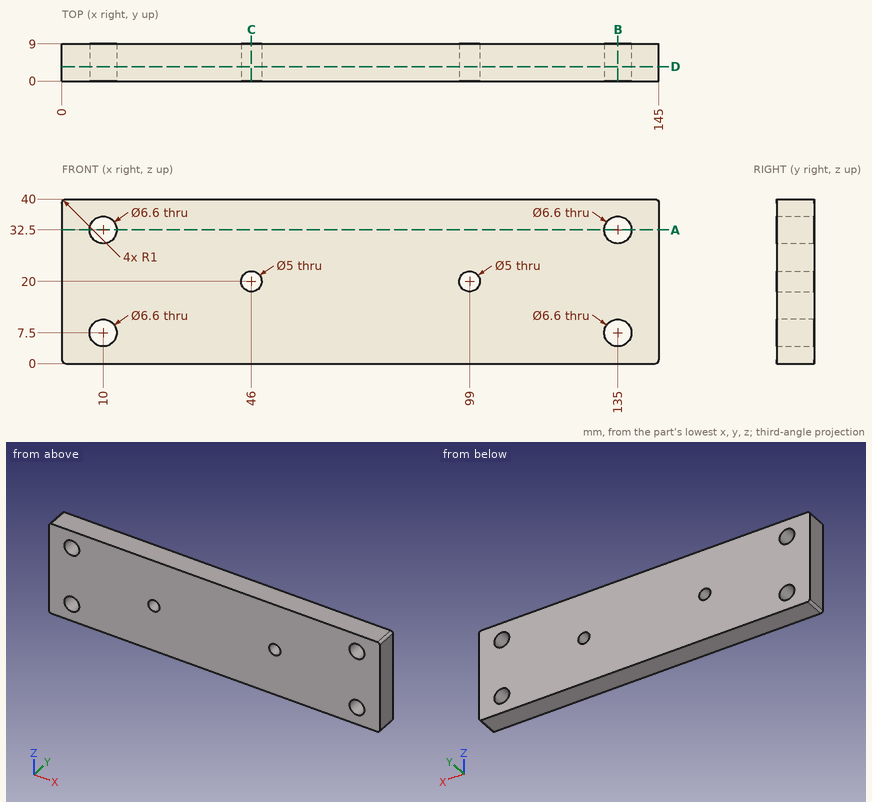
Source: three-view drawing plus pictorial views. Frame: mm from the lowest corner of the part. Give positions to 0.01 mm unless a question says otherwise; leave off trailing zeros. Order: outer loops, then holes, each group sorted by start corner. A loop starts at its lowest first (then second) coordinate and runs counter-clockwise, first axis right, second up. Notation, with made-up numbers: M 75.5,55 L 133.5,55 A23 cw 133.5,92 Z; hole C 4.5,72 d10. An arc over 180 degrees is marked long. One line per question, with ' | ' between items. Start each with the question number.
1. Section query B-B (x = 135). Return the cut outline in (y, z).
2. Section query C-C (x = 46). Return the cut outline in (y, z).
3. Material intervals for probe 1 along X at (y, z) = (3, 7.5); probe 2 along Z at (x, y) = (135, 3.5); probe 3 along X at (y, z) = (4.25, 20), sorted ascending. Write a range as [from, to].
4. Section query A-A (z = 32.5). Return the cut outline in (x, y), and give its area (3 significant figures).
5. Section query D-D (y = 3.5). Return the cut outline in (x, z), and give its area (3 significant figures).
Here are the results:
1) outline: M 0,0 L 9,0 L 9,4.2 L 0,4.2 Z; M 0,10.8 L 9,10.8 L 9,29.2 L 0,29.2 Z; M 0,35.8 L 9,35.8 L 9,40 L 0,40 Z
2) outline: M 0,0 L 9,0 L 9,17.5 L 0,17.5 Z; M 0,22.5 L 9,22.5 L 9,40 L 0,40 Z
3) probe 1: [0, 6.7], [13.3, 131.7], [138.3, 145] | probe 2: [0, 4.2], [10.8, 29.2], [35.8, 40] | probe 3: [0, 43.5], [48.5, 96.5], [101.5, 145]
4) outline: M 0,0 L 6.7,0 L 6.7,9 L 0,9 Z; M 13.3,0 L 131.7,0 L 131.7,9 L 13.3,9 Z; M 138.3,0 L 145,0 L 145,9 L 138.3,9 Z | area: 1,190 mm²
5) outline: M 0,1 A1 ccw 1,0 L 144,0 A1 ccw 145,1 L 145,39 A1 ccw 144,40 L 1,40 A1 ccw 0,39 Z; hole C 10,7.5 d6.6; hole C 10,32.5 d6.6; hole C 46,20 d5; hole C 99,20 d5; hole C 135,7.5 d6.6; hole C 135,32.5 d6.6 | area: 5,620 mm²
